Geometry: see drawing. Coordinates: mm, zero at the bounding-box minimum. A direction names the side the tool comes from. Round coordinates to 2 decimals unless told otherwise and drop trailing zeros. Order: outer loops, then holes, each group sorted by start corner. A loop starts at its lowest first (then second) coordinate and runs counter-clockwise, first axis right, second up. Notation, with made-up numbers: (37, 36) -> (76, 36) arc R31 ccw to (76, 63) -> close; hole circle Ø4 at (71.25, 23.25). An arc over 180 degrees is marked (long way). Answer as CSV lines item,"result". Start each with the question number.
(1) Line query: line 1 along Z through (x, y) = (16, 1.3); line 2 along Y through (x, z) = (30.6, 22.5); line 3 along Z through (x, y) = (29.1, 18). Output: solid intervals per line, ascending. Write a range as from..to.
(2) Contact query for flat-ended pins moving along their axis: P1, Ø4.5, axis at x = 16, z = 22.5, coming from the +Y side; P2, Ø10, axis at x = 20, z = 5, coming from the -Y side. Output: stop coordinate, or through.
(3) Section query A-A (x = 16). Output: boundary loops of the cut face in (y, z), plus the area to 3 significant figures.
(4) Section query C-C (z = 22.5). Output: boundary loops of the cut face in (x, y).
(5) Section query B-B (y = 18). Output: boundary loops of the cut face in (x, z).
(6) Set-up query: the marked faces 4 and 5. Return all of +Z, -Z, +X, -X, +Y, -Y with unobstructed straight access to the full face (end or side cutting, diameter ignored); none if empty.
(7) Section query D-D (y = 27). Output: boundary loops of the cut face in (x, z).
(8) Pull-direction query (X, two-part tool) for the marked faces 1, 2 and 3; classes: +X half, -X half, draft (parallel to the pull), parting line (faces both ways), or undercut.
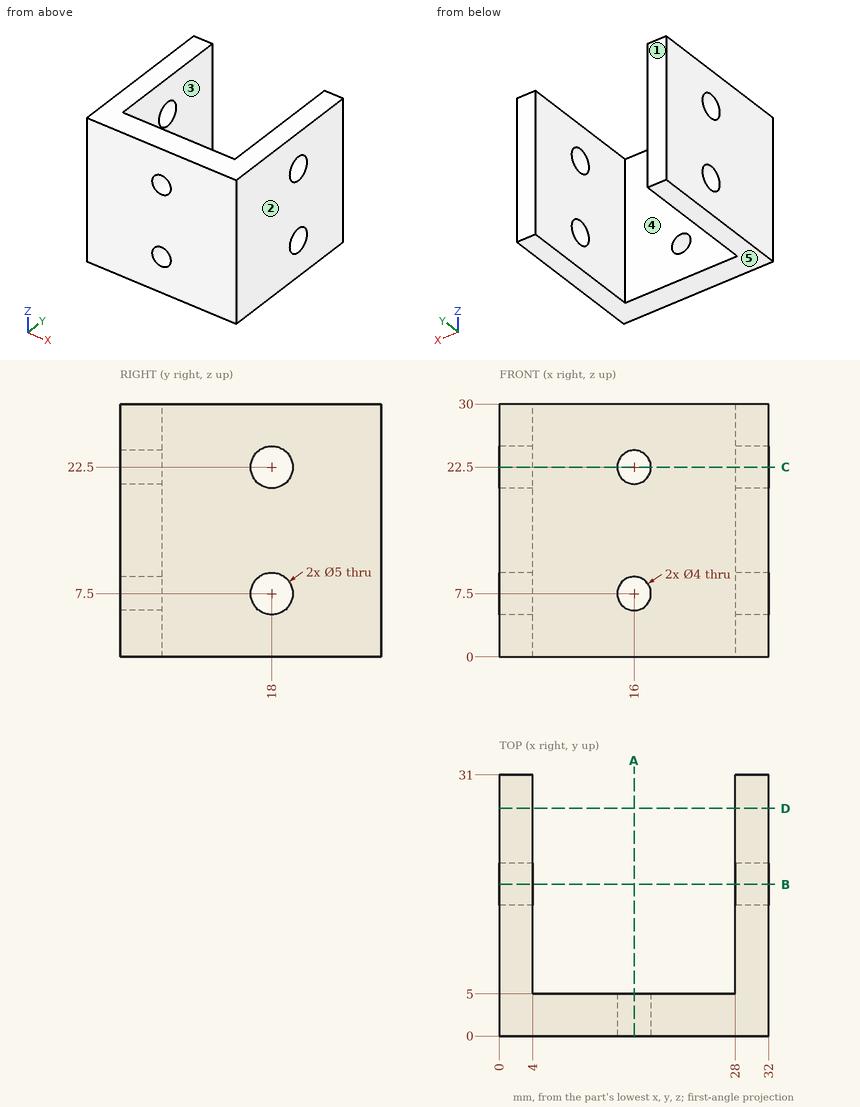
Answer block:
1,line 1,"0..5.5, 9.5..20.5, 24.5..30"
1,line 2,"0..15.5, 20.5..31"
1,line 3,"0..5, 10..20, 25..30"
2,P1,"y = 5"
2,P2,"y = 0"
3,outline,"(0, 0) -> (5, 0) -> (5, 5.5) -> (0, 5.5) -> close; (0, 9.5) -> (5, 9.5) -> (5, 20.5) -> (0, 20.5) -> close; (0, 24.5) -> (5, 24.5) -> (5, 30) -> (0, 30) -> close"
3,area,"110 mm2"
4,outline,"(0, 0) -> (14, 0) -> (14, 5) -> (4, 5) -> (4, 15.5) -> (0, 15.5) -> close; (0, 20.5) -> (4, 20.5) -> (4, 31) -> (0, 31) -> close; (18, 0) -> (32, 0) -> (32, 15.5) -> (28, 15.5) -> (28, 5) -> (18, 5) -> close; (28, 20.5) -> (32, 20.5) -> (32, 31) -> (28, 31) -> close"
5,outline,"(0, 0) -> (4, 0) -> (4, 5) -> (0, 5) -> close; (0, 10) -> (4, 10) -> (4, 20) -> (0, 20) -> close; (0, 25) -> (4, 25) -> (4, 30) -> (0, 30) -> close; (28, 0) -> (32, 0) -> (32, 5) -> (28, 5) -> close; (28, 10) -> (32, 10) -> (32, 20) -> (28, 20) -> close; (28, 25) -> (32, 25) -> (32, 30) -> (28, 30) -> close"
6,face 4,"+Z, -Z, +Y"
6,face 5,"-Z, +X, -X, +Y, -Y"
7,outline,"(0, 0) -> (4, 0) -> (4, 30) -> (0, 30) -> close; (28, 0) -> (32, 0) -> (32, 30) -> (28, 30) -> close"
8,face 1,"draft"
8,face 2,"+X half"
8,face 3,"undercut"
